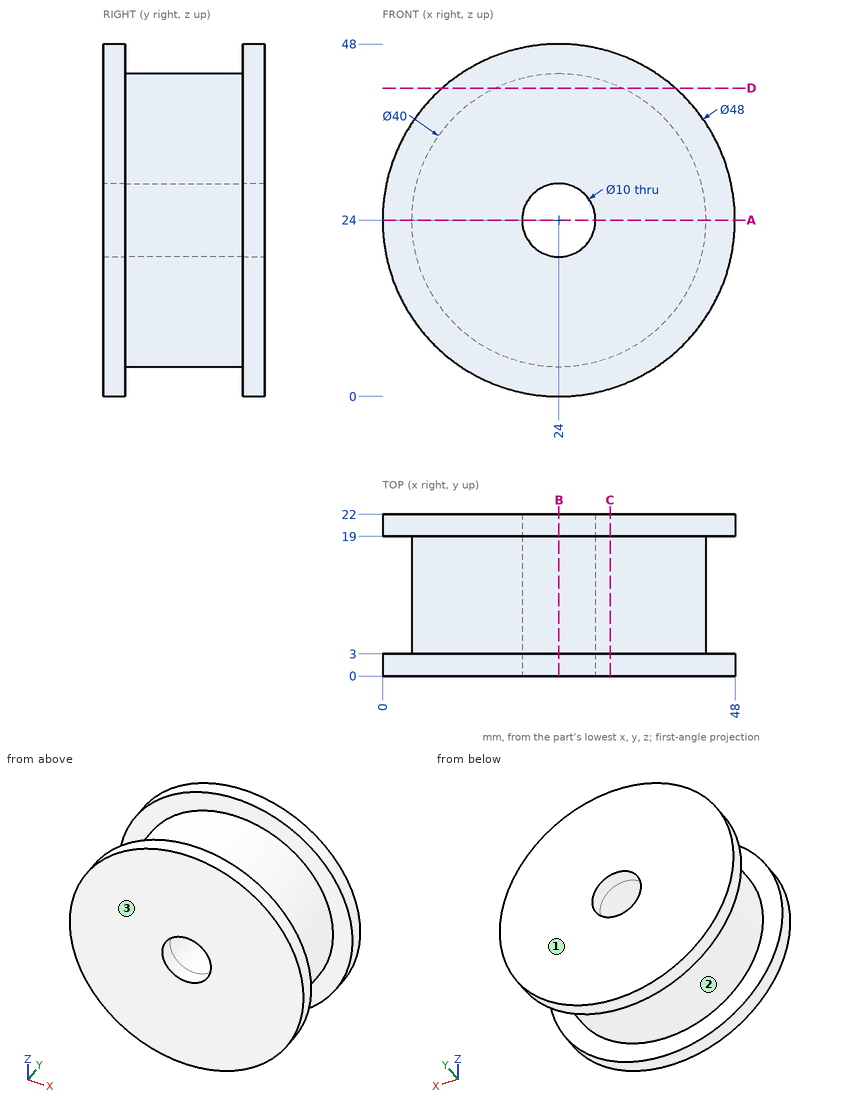
For this review, use the dimensioned drawing (mm, ordinates from the lowest corner) and the shaded views. Give positions to 0.01 mm unless a question says otherwise; leave off trailing zeros. Loops run counter-clockwise (first coordinate to the right, second up) from the corner with the lowest first, then second, coordinate; pieces in that order, holes last. Notation, with made-up numbers: (-30.5, 19) - (-12.5, 19) arc R32 ccw to (-12.5, 54) - close; hole circle Ø9 at (40.25, 81.5). An arc over 180 degrees is marked (long way). Write each question's results on one line, items separated by ' | '.
(1) Take a section at B-B (x = 24). Give the boundary of the cut face in (y, z), then the cut area to 3 significant figures.
Conclusion:
outline: (0, 0) - (3, 0) - (3, 4) - (19, 4) - (19, 0) - (22, 0) - (22, 19) - (0, 19) - close; (0, 29) - (22, 29) - (22, 48) - (19, 48) - (19, 44) - (3, 44) - (3, 48) - (0, 48) - close | area: 708 mm^2
(2) Take a section at A-A (z = 24). Give the boundary of the cut face in (x, y), then the cut area to 3 significant figures.
Conclusion:
outline: (0, 0) - (19, 0) - (19, 22) - (0, 22) - (0, 19) - (4, 19) - (4, 3) - (0, 3) - close; (29, 0) - (48, 0) - (48, 3) - (44, 3) - (44, 19) - (48, 19) - (48, 22) - (29, 22) - close | area: 708 mm^2
(3) For pin 1 Ø12 at (y, z) = (13.5, 29.5) entering from +X; pin 2 Ø4 at (y, z) = (5.5, 10) entering from -X; pin 3 Ø8 at (x, y) = (27, 11) entering from -Z; pin 4 Ø9 at (x, z) = (24, 24) entering from -Y, all flat-tipped, find the tip position at first contact; note any pin that passes through.
Conclusion:
pin 1: x = 47.8 | pin 2: x = 8 | pin 3: z = 4 | pin 4: through
(4) Take a section at C-C (x = 31). Give the boundary of the cut face in (y, z) (3 decimals).
Conclusion:
outline: (0, 1.044) - (3, 1.044) - (3, 5.265) - (19, 5.265) - (19, 1.044) - (22, 1.044) - (22, 46.956) - (19, 46.956) - (19, 42.735) - (3, 42.735) - (3, 46.956) - (0, 46.956) - close
(5) For line 1 along X through (y, z) = (15.75, 24); line 2 along X through (y, z) = (20.3, 24); line 3 along Z through (x, y) = (24.5, 7.25), list the stretches that pass through material, from the lowest coordinate up.
Conclusion:
line 1: 4 to 19, 29 to 44 | line 2: 0 to 19, 29 to 48 | line 3: 4.01 to 19.03, 28.97 to 43.99
(6) Take a section at D-D (z = 42). Give the boundary of the cut face in (x, y), then the cut area to 3 significant figures.
Conclusion:
outline: (8.13, 0) - (39.87, 0) - (39.87, 3) - (32.72, 3) - (32.72, 19) - (39.87, 19) - (39.87, 22) - (8.13, 22) - (8.13, 19) - (15.28, 19) - (15.28, 3) - (8.13, 3) - close | area: 469 mm^2
(7) Draft analysis for pull direction Y (two halves, no side actions). For the marked faces 1, 2 and 3, state which applies: +Y half, -Y half, draft (parallel to the pull), parting line (faces both ways), or undercut.
Conclusion:
face 1: +Y half | face 2: undercut | face 3: -Y half
